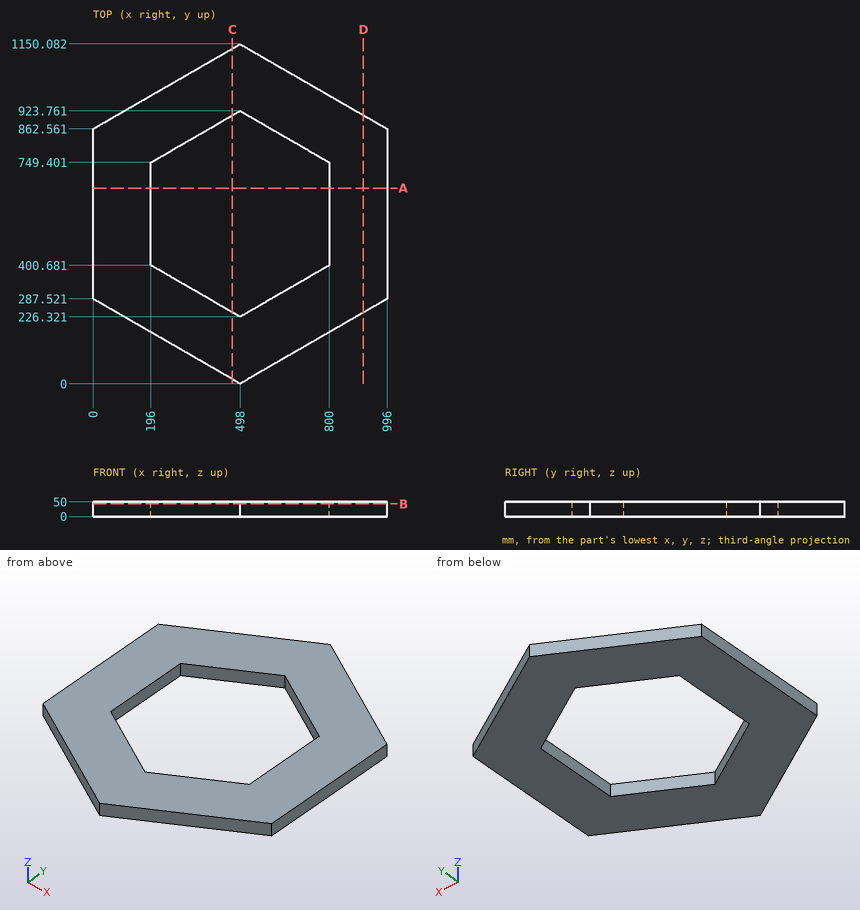
Can you work these out from the drawing? Everything is in mm from the part's minimum corner. Round coordinates to 2 decimals unless told otherwise and drop trailing zeros. Loops run counter-clockwise (first coordinate to the right, second up) from the corner with the lowest first, then second, coordinate; pieces in that order, holes last.
1. If we section it at A-A on y = 662: Write out the boundary of the cut face in (x, z).
Answer list:
outline: (0, 0) - (196, 0) - (196, 50) - (0, 50) - close; (800, 0) - (996, 0) - (996, 50) - (800, 50) - close
2. For P1, Ø4, axis at x = 727, z = 5.5, coming from the -Y side; P2, Ø1, axis at x = 325, z = 12, coming from the -Y side; P3, Ø1.5, axis at x = 731, z = 37, coming from the +Y side, each with a flat end and sliding along its axis, tell me the tip position at first contact or that it passes through.
Answer list:
P1: stops at y = 131.06
P2: stops at y = 99.59
P3: stops at y = 1015.99
3. If we section it at B-B on z = 42.5: Write out the boundary of the cut face in (x, y).
Answer list:
outline: (0, 287.52) - (498, 0) - (996, 287.52) - (996, 862.56) - (498, 1150.08) - (0, 862.56) - close; hole (196, 400.68) - (498, 226.32) - (800, 400.68) - (800, 749.4) - (498, 923.76) - (196, 749.4) - close
4. If I drill on line 1 along X through (y, z) = (457.5, 33.5); line 2 along X through (y, z) = (837, 20) (1 decimal); line 3 along Y through (x, z) = (577, 32.5), over which ranges is the centre line in solid material (lowest first)?
Answer list:
line 1: x = 0 to 196, 800 to 996
line 2: x = 0 to 347.7, 648.3 to 996
line 3: y = 45.61 to 271.93, 878.15 to 1104.47
5. If we section it at D-D on x = 915: Write out the boundary of the cut face in (y, z) (1 decimal), plus the area to 3 significant figures.
Answer list:
outline: (240.8, 0) - (909.3, 0) - (909.3, 50) - (240.8, 50) - close
area: 33,400 mm2
6. If we section it at C-C on x = 471.5: Write out the boundary of the cut face in (y, z), plus the area to 3 significant figures.
Answer list:
outline: (15.3, 0) - (241.62, 0) - (241.62, 50) - (15.3, 50) - close; (908.46, 0) - (1134.78, 0) - (1134.78, 50) - (908.46, 50) - close
area: 22,600 mm2
